Can you work these out from the model? Positions are in its coordinate system, mm. Face numbers are marked on the shaded views. Round coordinates to 2 decimals unless told otherwise and drop trailing zeros. Loops run counter-clockwise (first coordinate to the right, second up) from the corner with the lowest first, then second, coordinate; pieces in that order, holes last. Notation, with made-up numbers: (74, 1) - (120, 1) arc R11 cw to (120, 21) - close; hole circle Ø9 at (1, -27.75). An arc over 180 degrees is marked (long way). Answer as CSV lines item,"result".
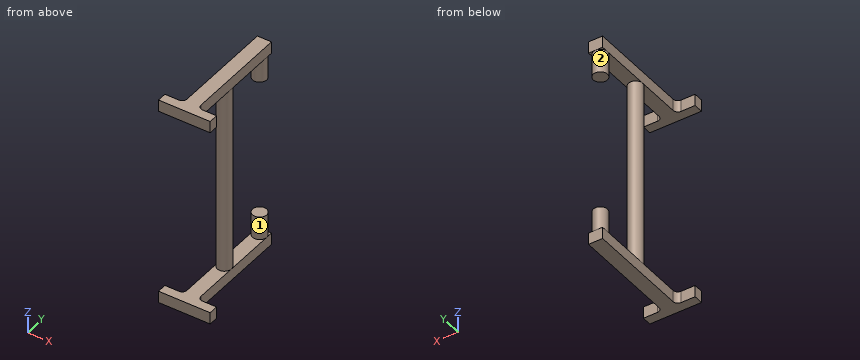
```python
from build123d import *

# Parameters (mm, degrees)
SKETCH1_R            = 3
BOSS_EXTRUDE1_DEPTH  = 40
SKETCH2_W            = 6
SKETCH2_H            = 50
BOSS_EXTRUDE2_DEPTH  = 5
SKETCH9_W            = 22
SKETCH9_H            = 5
BOSS_EXTRUDE5_DEPTH  = 4
FILLET1_R            = 2
SKETCH11_R           = 3
BOSS_EXTRUDE7_DEPTH  = 10
FILLET1_OF_MIRROR5_R = 2


with BuildPart() as part:
    # Sketch1 → Boss-Extrude1 (new, symmetric)
    with BuildSketch(Plane.XY):
        Circle(SKETCH1_R)
    extrude(amount=BOSS_EXTRUDE1_DEPTH, both=True)

    # Sketch2 → Boss-Extrude2 (add)
    with BuildSketch(Plane.XY.offset(40)):
        Rectangle(SKETCH2_W, SKETCH2_H)
    boss_extrude2 = extrude(amount=BOSS_EXTRUDE2_DEPTH)

    # Sketch9 → Boss-Extrude5 (add)
    with BuildSketch(Plane.XZ.offset(25)):
        with Locations((0, 42.5)):
            Rectangle(SKETCH9_W, SKETCH9_H)
    boss_extrude5 = extrude(amount=-BOSS_EXTRUDE5_DEPTH)

    # Fillet1
    fillet1_edges = [part.edges().sort_by_distance(p)[0] for p in [
        (-3, -21, 42.5),
        (3, -21, 42.5),
    ]]
    fillet(fillet1_edges, radius=FILLET1_R)

    # Sketch11 → Boss-Extrude7 (add)
    with BuildSketch(Plane(origin=(0, 0, 40), x_dir=(-1, 0, 0), z_dir=(0, 0, -1))):
        with Locations((0, 22)):
            Circle(SKETCH11_R)
    boss_extrude7 = extrude(amount=BOSS_EXTRUDE7_DEPTH)

    # Mirror5: Boss-Extrude2, Boss-Extrude5, Boss-Extrude7 across plane
    add(boss_extrude2.mirror(Plane.XY))
    add(boss_extrude5.mirror(Plane.XY))
    add(boss_extrude7.mirror(Plane.XY))

    # Fillet1 of Mirror5
    fillet1_of_mirror5_edges = [part.edges().sort_by_distance(p)[0] for p in [
        (-3, -21, -42.5),
        (3, -21, -42.5),
    ]]
    fillet(fillet1_of_mirror5_edges, radius=FILLET1_OF_MIRROR5_R)

    # Mirror1: Boss-Extrude2 across plane
    add(boss_extrude2.mirror(Plane.XY))


solid = part.part
```
Q1. Imagine slicing it at D-D (z = 21). Write out the boundary of the cut face in (x, y).
Checks:
outline,"circle Ø6 at (0, 0)"
Q2. Imagine slicing it at B-B (x = -9.5). Write out the boundary of the cut face in (y, z), then the cut area to 3 significant figures.
Checks:
outline,"(-25, -45) - (-21, -45) - (-21, -40) - (-25, -40) - close; (-25, 40) - (-21, 40) - (-21, 45) - (-25, 45) - close"
area,"40.0 mm²"
Q3. Imagine slicing it at A-A (y = 15.5). Write out the boundary of the cut face in (x, z).
Checks:
outline,"(-3, -45) - (3, -45) - (3, -40) - (-3, -40) - close; (-3, 40) - (3, 40) - (3, 45) - (-3, 45) - close"
Q4. We'd pull the mould along Y, two halves only. Please class the marked faces 1 and 2: pulls with the +Y half, pulls with the -Y half, needs draft (parallel to the pull), parting line crosses it, or undercut.
Checks:
face 1,"undercut"
face 2,"undercut"
Q5. I'm going to push flat-ended pins straight in: pin 1 Ø6 at (x, z) = (5.5, -24.5) entering from +Y; pin 2 Ø5.5 at (x, z) = (-7.5, -43.5) entering from +Y; pin 3 Ø1.5 at (x, z) = (-3.5, 32) entering from -Y. Where does each tip first touch, or does it pass through?
Checks:
pin 1,"y = 1.66"
pin 2,"y = -20.98"
pin 3,"y = -1.2"
Q6. Imagine slicing it at C-C (z = 35). Write out the boundary of the cut face in (x, y).
Checks:
outline,"circle Ø6 at (0, 0); circle Ø6 at (0, 22)"
Q7. If I drill on line 1 along Z through (x, y) = (-9, -21.5); line 2 along Z through (x, y) = (-1.5, 22); line 3 along X through (y, z) = (15.5, 40.5), over which ranges is the centre line in solid material (lowest first)? Write a range as [from, to].
Checks:
line 1,"[-45, -40], [40, 45]"
line 2,"[-45, -30], [30, 45]"
line 3,"[-3, 3]"
